The listing builds one solid part. Answer for the finished solid, in the listing's coordinates (mm). Coordinates: 2 decimals unless noted, no trailing zeros. Order: outer loops, then holes, each group sorted by start corner. A loop starts at its lowest first (then second) coordinate and runs counter-clockwise, first axis right, second up. Notation, with made-up numbers: M 28,80 L 83,80 A13 cw 83,99 Z; hole C 6.5,16.5 d6. An arc over 180 degrees is marked long. One line per item, written item: value. Start each with the question number.
Q1. The part is cut by section A-A on z = 35. Give the vertices of the cut face in (x, y).
Q2. The part is cut by section B-B on y = -2.5. Give the vertices of the cut face in (x, z).
Q3. Straight lines are drawn through the part: line 1 along Y through (x, z) = (-73.5, 44); line 2 along X through (y, z) = (-38, 56); line 3 along Z through (x, y) = (-73, 13.5). For each, find the intervals that lie inside material, in ascending order. Write a range as [from, to].
Q4. Each of these flat-tipped pins is pushed along its axis until it touches: pin 1 Ø1.5 at (x, z) = (-76.5, 36.5) entering from +Y; pin 2 Ø2.5 at (x, y) = (-76, 11) entering from +Z; pin 3 Ø1.5 at (y, z) = (-1, 3.5) entering from +X. Where does it stop, or does it pass through?
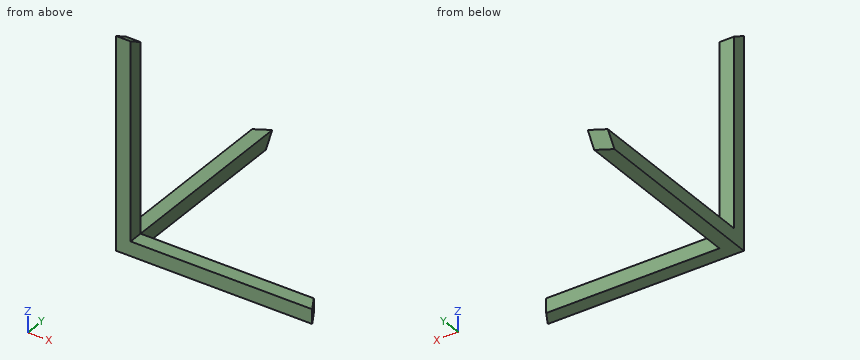
```python
from build123d import *

# Parameters (mm, degrees)
SKETCH1_W           = 5
SKETCH1_H           = 65
BOSS_EXTRUDE1_DEPTH = 5
SKETCH2_W           = 65
SKETCH2_H           = 5
BOSS_EXTRUDE3_DEPTH = 5
SKETCH4_W           = 65
SKETCH4_H           = 5
BOSS_EXTRUDE4_DEPTH = 5
DRAFT3_ANGLE        = 30
DRAFT7_ANGLE        = 30
DRAFT8_ANGLE        = 30
DRAFT9_ANGLE        = 30


with BuildPart() as part:
    # Sketch1 → Boss-Extrude1 (new body)
    with BuildSketch(Plane.XY):
        with Locations((-75.007440829, -10.132080835)):
            Rectangle(SKETCH1_W, SKETCH1_H)
    extrude(amount=BOSS_EXTRUDE1_DEPTH)

    # Sketch2 → Boss-Extrude3 (add)
    with BuildSketch(Plane.ZY.offset(77.507440829)):
        with Locations((37.5, -40.132080835)):
            Rectangle(SKETCH2_W, SKETCH2_H)
    extrude(amount=-BOSS_EXTRUDE3_DEPTH)

    # Sketch4 → Boss-Extrude4 (add)
    with BuildSketch(Plane(origin=(0, -37.632080835, 0), x_dir=(1, 0, 0), z_dir=(0, 1, 0))):
        with Locations((-45.007440829, -2.5)):
            Rectangle(SKETCH4_W, SKETCH4_H)
    extrude(amount=-BOSS_EXTRUDE4_DEPTH)

    # Draft3
    draft3_faces = [part.faces().sort_by_distance(p)[0] for p in [
        (-12.507440829, -40.132080835, 2.5),
    ]]
    draft(draft3_faces, Plane.ZX.offset(-37.632080835), DRAFT3_ANGLE)

    # Draft7
    draft7_faces = [part.faces().sort_by_distance(p)[0] for p in [
        (-75.007440829, -40.132080835, 70),
    ]]
    draft(draft7_faces, Plane(origin=(-72.507440829, -37.632080835, 5), x_dir=(0, 0, 1), z_dir=(0, 1, 0)), DRAFT7_ANGLE)

    # Draft8
    draft8_faces = [part.faces().sort_by_distance(p)[0] for p in [
        (-75.007440829, 22.367919165, 2.5),
    ]]
    draft(draft8_faces, Plane(origin=(-77.507440829, 22.367919165, 5), x_dir=(0, 0, -1), z_dir=(-1, 0, 0)), DRAFT8_ANGLE)

    # Draft9
    draft9_faces = [part.faces().sort_by_distance(p)[0] for p in [
        (-75.007440829, 23.811294838, 2.5),
    ]]
    draft(draft9_faces, Plane(origin=(0, 0, 0), x_dir=(-1, 0, 0), z_dir=(0, 0, -1)), DRAFT9_ANGLE)


solid = part.part
```
Output:
1. outline: M -77.51,-42.63 L -72.51,-42.63 L -72.51,-37.63 L -77.51,-37.63 Z
2. outline: M -77.51,0 L -72.51,0 L -72.51,5 L -77.51,5 Z
3. line 1: y = [-42.63, -37.63]
3. line 2: x = [-77.51, -72.51]
3. line 3: z = [0, 5]
4. pin 1: stops at y = -37.63
4. pin 2: stops at z = 5
4. pin 3: stops at x = -72.51
